The listing builds one solid part. Answer for the finished solid, in the listing's coordinates (mm). Coordinates: 2 decimals unless noted, no trailing zeros. Write each loop counter-clockwise with the first axis right and the second up, starting at its lowest first coordinate (ties: lowest second). Pieces come first, ordered by that corner, then holes.
from build123d import *

# Parameters (mm, degrees)
PAD021_DEPTH                        = 3
SKETCH083_R                         = 1.7
POCKET041_DEPTH                     = 0.001
POCKET041_DEPTH_BACK                = 3.001
SKETCH084_R                         = 1.7
POCKET042_DEPTH                     = 0.001
POCKET042_DEPTH_BACK                = 3.001
BODY001003005003013_PLACEMENT_ANGLE = 60
CLONE017_PLACEMENT_ANGLE            = 58


with BuildPart() as part:
    # Sketch082 → Pad021 (new body)
    with BuildSketch(Plane.XY):
        with BuildLine():
            ThreePointArc((156.627412, 120.879551), (87.258751, 177.56667), (0, 197.848457))
            Line((0, 197.848457), (0, 182.848457))
            ThreePointArc((144.752611, 111.714995), (80.643177, 164.104346), (0, 182.848457))
            ThreePointArc((148.102078, 107.234942), (146.444477, 109.487778), (144.752611, 111.714995))
            ThreePointArc((148.102078, 107.234942), (148.703343, 106.843433), (149.41205, 106.955386))
            Line((155.154429, 110.27075), (149.41205, 106.955386))
            Line((155.154429, 110.27075), (160.726477, 113.487773))
            ThreePointArc((160.726477, 113.487773), (161.203737, 114.141753), (161.040435, 114.934722))
            ThreePointArc((161.040435, 114.934722), (158.861734, 117.927781), (156.627412, 120.879551))
        make_face()
    pad021 = extrude(amount=PAD021_DEPTH)

    # Mirrored029: Pad021 across Sketch082 V_Axis
    add(pad021.mirror(Plane(origin=(0, 0, 0), x_dir=(0, 0, 1), z_dir=(1, 0, 0))))

    # Sketch083 → Pocket041 (cut, two sides)
    with BuildSketch(Plane.XY) as pocket041_sk:
        with Locations((149.149219, 118.266841)):
            Circle(SKETCH083_R)
        with Locations((-149.149219, 118.266841)):
            Circle(SKETCH083_R)
    extrude(amount=-POCKET041_DEPTH, mode=Mode.SUBTRACT)
    extrude(pocket041_sk.sketch, amount=POCKET041_DEPTH_BACK, mode=Mode.SUBTRACT)

    # Sketch084 → Pocket042 (cut, two sides)
    with BuildSketch(Plane.XY) as pocket042_sk:
        with Locations((0, 190.348457)):
            Circle(SKETCH084_R)
    extrude(amount=-POCKET042_DEPTH, mode=Mode.SUBTRACT)
    extrude(pocket042_sk.sketch, amount=POCKET042_DEPTH_BACK, mode=Mode.SUBTRACT)


with BuildPart() as part_1:
    # Body001003005003013 placement: moved
    add(part.part.rotate(Axis((0, 0, 0), (0, 0, 1)), BODY001003005003013_PLACEMENT_ANGLE))


with BuildPart() as part_2:
    # Clone017 placement: moved
    add(part_1.part.moved(Location((817, 805, 0))).rotate(Axis((817, 805, 0), (0, 0, -1)), CLONE017_PLACEMENT_ANGLE))


solid = part_2.part
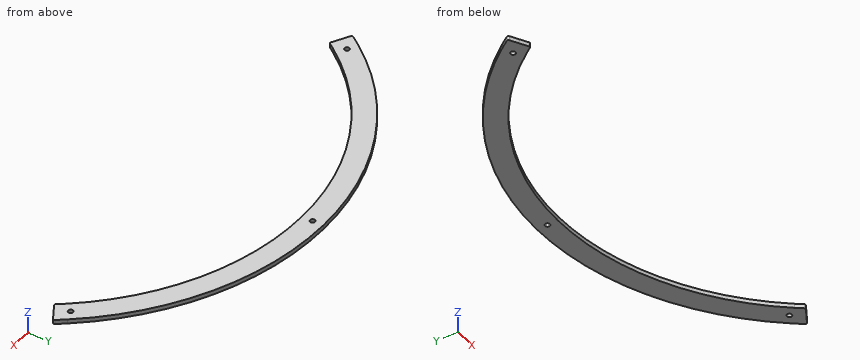
1. Section D-D on x = 702.5 is taken. Give the vertices of the cut face in (y, z).
Results found:
outline: (947.56, 0) - (966.35, 0) - (966.35, 3) - (947.56, 3) - close
2. Section B-B on z = 2.1 is taken. Give the vertices of the cut face in (x, y).
Results found:
outline: (652.05, 914.24) arc R1 ccw to (652.41, 912.81) - (663.95, 906.68) arc R1 ccw to (665.25, 907) arc R182.85 cw to (668.44, 911.6) arc R182.85 cw to (810.62, 987.74) arc R182.85 cw to (957.77, 921.7) arc R182.85 cw to (961.27, 917.34) arc R1 ccw to (962.59, 917.1) - (973.67, 924.03) arc R1 ccw to (973.93, 925.48) arc R197.85 ccw to (969.31, 931.27) arc R197.85 ccw to (656.25, 920.34) arc R197.85 ccw to start; hole circle Ø3.4 at (663.81, 917.99); hole circle Ø3.4 at (810.36, 995.23); hole circle Ø3.4 at (961.93, 928.4)
3. Flat-ended cylindrical pins translate along their axes: P1, Ø2.5, axis at x = 663.81, y = 917.99, coming from the -Z side; P2, Ø1.5, axis at x = 725, z = 2, coming from the +Y side; P3, Ø4, axis at x = 700.5, y = 965.5, coming from the -Z side; P4, Ø1, axis at x = 893, z = 2, coming from the -Y side. Find the tip coordinate at first contact, or state that the pin passes through.
Results found:
P1: passes through
P2: stops at y = 980.55
P3: stops at z = 0
P4: stops at y = 971.08
4. Find the intervals of material crossed by L1, parallel to X at y = 971, z = 1.6; L2, parallel to X at y = 926, z = 2.7; L3, parallel to Y at x = 708.5, z = 1.05, in increasing order.
Results found:
L1: x = 709.35 to 740.33, 893.67 to 924.65
L2: x = 660.47 to 679.91, 954.09 to 973.53
L3: y = 952.18 to 970.44
5. Section C-C on y = 942 is taken. Give the vertices of the cut face in (x, z).
Results found:
outline: (674.26, 0) - (695.9, 0) - (695.9, 3) - (674.26, 3) - close; (938.1, 0) - (959.74, 0) - (959.74, 3) - (938.1, 3) - close
6. Section A-A on y = 980 is taken. Give the vertices of the cut face in (x, z).
Results found:
outline: (724.7, 0) - (764, 0) - (764, 3) - (724.7, 3) - close; (870, 0) - (909.3, 0) - (909.3, 3) - (870, 3) - close
